from build123d import *

# Parameters (mm, degrees)
ESQUISSE1_W             = 120
ESQUISSE1_H             = 65
ESQUISSE1_R             = 6.25
BOSS_EXTRU_1_DEPTH      = 5
ESQUISSE2_W             = 120
ESQUISSE2_H             = 65
ESQUISSE2_W_2           = 110
ESQUISSE2_H_2           = 55
BOSS_EXTRU_3_DEPTH      = 45
ESQUISSE4_W             = 120
ESQUISSE4_H             = 65
BOSS_EXTRU_4_DEPTH      = 5
ESQUISSE5_W             = 55
ESQUISSE5_H             = 65
ENL_V_MAT_EXTRU_1_DEPTH = 5
ESQUISSE6_W             = 2
ESQUISSE6_H             = 61
ENL_V_MAT_EXTRU_2_DEPTH = 62.25
BOSS_EXTRU_6_DEPTH      = 110
ESQUISSE8_R             = 3
ENL_V_MAT_EXTRU_3_DEPTH = 12
ESQUISSE9_R             = 4.6
ENL_V_MAT_EXTRU_7_DEPTH = 1.5


with BuildPart() as part:
    # Esquisse1 → Boss.-Extru.1 (new body)
    with BuildSketch(Plane.XY):
        with Locations((60, 32.5)):
            Rectangle(ESQUISSE1_W, ESQUISSE1_H)
        with Locations((30, 32.5)):
            Circle(ESQUISSE1_R, mode=Mode.SUBTRACT)
        with Locations((90, 32.5)):
            Circle(ESQUISSE1_R, mode=Mode.SUBTRACT)
    extrude(amount=BOSS_EXTRU_1_DEPTH)

    # Esquisse2 → Boss.-Extru.3 (add)
    with BuildSketch(Plane.XY.offset(5)):
        with Locations((60, 32.5)):
            Rectangle(ESQUISSE2_W, ESQUISSE2_H)
        with Locations((60, 32.5)):
            Rectangle(ESQUISSE2_W_2, ESQUISSE2_H_2, mode=Mode.SUBTRACT)
    extrude(amount=BOSS_EXTRU_3_DEPTH)

    # Esquisse4 → Boss.-Extru.4 (add)
    with BuildSketch(Plane.XY.offset(50)):
        with Locations((60, 32.5)):
            Rectangle(ESQUISSE4_W, ESQUISSE4_H)
    extrude(amount=BOSS_EXTRU_4_DEPTH)

    # Esquisse5 → Enlèv. mat.-Extru.1 (cut)
    with BuildSketch(Plane(origin=(120, 0, 0), x_dir=(0, 0, -1), z_dir=(1, 0, 0))):
        with Locations((-27.5, 32.5)):
            Rectangle(ESQUISSE5_W, ESQUISSE5_H)
    extrude(amount=-ENL_V_MAT_EXTRU_1_DEPTH, mode=Mode.SUBTRACT)

    # Esquisse6 → Enlèv. mat.-Extru.2 (cut)
    with BuildSketch(Plane(origin=(115, 0, 0), x_dir=(0, 0, -1), z_dir=(1, 0, 0))):
        with Locations((-47, 32.5)):
            Rectangle(ESQUISSE6_W, ESQUISSE6_H)
    extrude(amount=-ENL_V_MAT_EXTRU_2_DEPTH, mode=Mode.SUBTRACT)

    # Esquisse7 → Boss.-Extru.6 (add)
    with BuildSketch(Plane(origin=(115, 0, 0), x_dir=(0, 0, -1), z_dir=(1, 0, 0))):
        with BuildLine():
            Line((-22.5, 60), (-32.5, 60))
            ThreePointArc((-32.5, 60), (-27.5, 55), (-22.5, 60))
        make_face()
        with BuildLine():
            Line((-32.5, 5), (-22.5, 5))
            ThreePointArc((-22.5, 5), (-27.5, 10), (-32.5, 5))
        make_face()
    extrude(amount=-BOSS_EXTRU_6_DEPTH)

    # Esquisse8 → Enlèv. mat.-Extru.3 (cut)
    with BuildSketch(Plane(origin=(115, 0, 0), x_dir=(0, 0, -1), z_dir=(1, 0, 0))):
        with Locations((-27.5, 60)):
            Circle(ESQUISSE8_R)
        with Locations((-27.5, 5)):
            Circle(ESQUISSE8_R)
    extrude(amount=-ENL_V_MAT_EXTRU_3_DEPTH, mode=Mode.SUBTRACT)

    # Esquisse9 → Enlèv. mat.-Extru.7 (cut)
    with BuildSketch(Plane(origin=(115, 0, 0), x_dir=(0, 0, -1), z_dir=(1, 0, 0))):
        with Locations((-27.5, 60)):
            Circle(ESQUISSE9_R)
        with Locations((-27.5, 5)):
            Circle(ESQUISSE9_R)
    extrude(amount=-ENL_V_MAT_EXTRU_7_DEPTH, mode=Mode.SUBTRACT)


solid = part.part
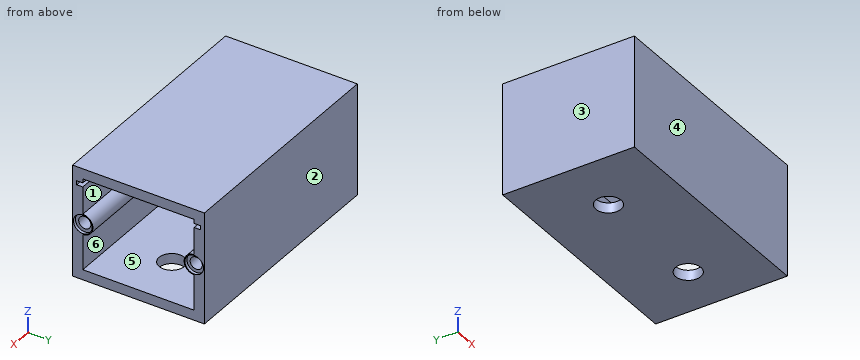
Work out the finished part from the listing and answer in its coordinate system (mm). Face numbers are marked on the shaded views. A direction names the side the tool comes from. Coordinates: 2 decimals unless noted, no trailing zeros. Loops run counter-clockwise (first coordinate to the right, second up) from the corner with the lowest first, then second, coordinate; pieces in that order, holes last. Notation, with made-up numbers: M -6,45.25 L 7,45.25 A19 ccw 7,51.25 Z; hole C 30.25,-17 d5. An arc over 180 degrees is marked long. Answer in a Markdown table with one row per item. Add a question column.
1. Find section A-A, the plane y = 32.5. Write down the section's boundary in (x, z).
2. Find section B-B, the plane x = 108.5. Write down the section's boundary in (y, z), then the cut area to 3 significant figures.
3. Flat-ended cylindrical pins translate along their axes: P1, Ø8.5, axis at y = 60, z = 27.5, coming from the -X side; P2, Ø3, axis at y = 4.5, z = 26, coming from the +X side; P3, Ø0.6, axis at y = 62, z = 47, coming from the +X side; P4, Ø11, axis at x = 90, y = 32.5, coming from the -Z side. Find the tip coordinate at first contact, or state that the pin passes through.
4. Find section C-C, the plane z = 27.5. Write down the section's boundary in (x, y).
5. Consider L1, parallel to Y at x = 114.3, z = 27.5; L2, parallel to Y at x = 48.5, z = 35; L3, parallel to Z at x = 110, y = 40. Determine where each line is inside the solid, lowest interval first.
6. A tool of negligible diameter and unlimited length cuts with its end or side. For the marked faces 1 and 2, from which of +Z, -Z, +X, -X, +Y, -Y can it reach the whole face along a straight path? Write none if from no direction.
7. The mould has two halves that part along Y. Classify the marked faces 3, 4, 5 and 6: pulls with the +Y half, pulls with the -Y half, needs draft (parallel to the pull), parting line crosses it, or undercut.
8. Find section D-D, the plane y = 43. Write down the section's boundary in (x, z), then the cut area to 4 significant figures.
Reported:
| question | item | result |
|---|---|---|
| 1 | outline | M 0,0 L 23.75,0 L 23.75,5 L 5,5 L 5,50 L 115,50 L 115,55 L 0,55 Z; M 36.25,0 L 83.75,0 L 83.75,5 L 36.25,5 Z; M 96.25,0 L 115,0 L 115,5 L 96.25,5 Z |
| 2 | outline | M 0,0 L 65,0 L 65,55 L 0,55 Z; hole C 5,27.5 d6; hole M 2,46 L 5,46 L 5,32.5 A5 cw 5,22.5 L 5,5 L 60,5 L 60,22.5 A5 cw 60,32.5 L 60,46 L 63,46 L 63,48 L 60,48 L 60,50 L 5,50 L 5,48 L 2,48 Z; hole C 60,27.5 d6 |
| 2 | area | 1,110 mm^2 |
| 3 | P1 | stops at x = 0 |
| 3 | P2 | stops at x = 113.5 |
| 3 | P3 | stops at x = 52.75 |
| 3 | P4 | stops at z = 50 |
| 4 | outline | M 0,0 L 115,0 L 115,0.4 L 113.5,0.4 L 113.5,2 L 103,2 L 103,8 L 113.5,8 L 113.5,9.6 L 115,9.6 L 115,10 L 5,10 L 5,55 L 115,55 L 115,55.4 L 113.5,55.4 L 113.5,57 L 103,57 L 103,63 L 113.5,63 L 113.5,64.6 L 115,64.6 L 115,65 L 0,65 Z |
| 5 | L1 | y = 0 to 0.4, 9.6 to 10, 55 to 55.4, 64.6 to 65 |
| 5 | L2 | y = 0 to 5, 60 to 65 |
| 5 | L3 | z = 0 to 5, 50 to 55 |
| 6 | face 1 | +X |
| 6 | face 2 | +Z, -Z, +X, -X, +Y |
| 7 | face 3 | needs draft |
| 7 | face 4 | pulls with the -Y half |
| 7 | face 5 | undercut |
| 7 | face 6 | undercut |
| 8 | outline | M 0,0 L 115,0 L 115,5 L 5,5 L 5,50 L 115,50 L 115,55 L 0,55 Z |
| 8 | area | 1,375 mm^2 |
